Read the model definition and answer for the solid it produces. Units are mm, in the model's axes. A direction names the side the tool comes from. Coordinates: 2 decimals unless noted, no trailing zeros. Write each loop counter-clockwise with the first axis right and the second up, starting at its lowest first coordinate (ties: lowest second). Pieces come first, ordered by that corner, then holes.
(1) Section A-A on y = -30.5 is taken. Write down the section's boundary in (x, z) (3 decimals).
(2) Given pin 1 (2 mm diameter, centred on y = 16, z = 15.5, fed in from +X); pin 2 (4 mm diameter, centred on x = -27.5, y = -8.5, fed in from +Z); pin 3 (5 mm diameter, centred on y = -14.5, z = -34, fed in from +X); pin 4 (21 mm diameter, centred on y = 8.5, z = -7.5, fed in from -X) (3 decimals), each flat-ended and moving along its own axis, determine where each tip first touches the part or whether it passes through.
(3) Which of the six approach directions +Z, -Z, +X, -X, +Y, -Y give full straight-line access (tool end or side, diameter ignored) to faces 5 (the cylindrical face through (20.882, -32.56, 13.314)), 6 (the cylindrical face through (-32.56, 13.314, 20.882)), 7 (the cylindrical face through (6.33, -20.11, -40.27))?
(4) Find the intervals of material crossed by probe 1 along X at (y, z) = (0, -39.5) (3 decimals); probe 2 along X at (y, z) = (0, -16.25) (3 decimals), in increasing order.
(5) The mould has two halves that part along X. Classify faces 1 (the conical face through (-20.755, -58.745, -4.609)), 2 (the cylindrical face through (-40.27, 20.11, 6.33)), 3 (the flat face through (16, 3, -20.955)), 4 (the cylindrical face through (10.73, 11.7, -12.95)): +X half, -X half, draft (parallel to the pull), parting line (faces both ways), or undercut.
from build123d import *


with BuildPart() as f3:
    # F0 (on Right) → F3 (revolve)
    with BuildSketch(Plane.YZ):
        with BuildLine():
            Line((-52.6758568757, 24.765), (-59.055, 21.082))
            Line((-59.055, 21.082), (-20.955, 21.082))
            Line((-20.955, 21.082), (-20.955, 15.875))
            Line((-20.955, 15.875), (0, 15.875))
            ThreePointArc((0, 15.875), (11.2253201513, 11.2253201513), (15.875, 0))
            Line((15.875, 0), (24.765, 0))
            ThreePointArc((24.765, 0), (17.5114994361, 17.5114994361), (0, 24.765))
            Line((0, 24.765), (-52.6758568757, 24.765))
        make_face()
        with BuildLine():
            Line((-20.955, 21.082), (-59.055, 21.082))
            Line((-59.055, 21.082), (-59.055, 0))
            Line((-59.055, 0), (0, 0))
            Line((0, 0), (10.5189766587, 0))
            Line((10.5189766587, 0), (15.875, 0))
            ThreePointArc((15.875, 0), (11.2253201513, 11.2253201513), (0, 15.875))
            Line((0, 15.875), (-20.955, 15.875))
            Line((-20.955, 15.875), (-20.955, 21.082))
        make_face()
    revolve(axis=Axis((0, -21.59, 0), (0, 1, 0)))

    # F1 (on Right) → F4 (revolve)
    with BuildSketch(Plane.YZ):
        with BuildLine():
            Line((-24.765, -52.6758568757), (-21.082, -59.055))
            Line((-21.082, -59.055), (-21.082, -20.955))
            Line((-21.082, -20.955), (-15.875, -20.955))
            Line((-15.875, -20.955), (-15.875, 0))
            ThreePointArc((-15.875, 0), (-11.2253201513, 11.2253201513), (0, 15.875))
            Line((0, 15.875), (0, 24.765))
            ThreePointArc((0, 24.765), (-17.5114994361, 17.5114994361), (-24.765, 0))
            Line((-24.765, 0), (-24.765, -52.6758568757))
        make_face()
        with BuildLine():
            Line((-21.082, -20.955), (-21.082, -59.055))
            Line((-21.082, -59.055), (0, -59.055))
            Line((0, -59.055), (0, 0))
            Line((0, 0), (0, 15.875))
            ThreePointArc((0, 15.875), (-11.2253201513, 11.2253201513), (-15.875, 0))
            Line((-15.875, 0), (-15.875, -20.955))
            Line((-15.875, -20.955), (-21.082, -20.955))
        make_face()
    revolve(axis=Axis((0, 0, -21.59), (0, 0, 1)))

    # F2 (on Top) → F5 (revolve)
    with BuildSketch(Plane.XY):
        with BuildLine():
            Line((-52.6758568757, 24.765), (-59.055, 21.082))
            Line((-59.055, 21.082), (-20.955, 21.082))
            Line((-20.955, 21.082), (-20.955, 15.875))
            Line((-20.955, 15.875), (0, 15.875))
            ThreePointArc((0, 15.875), (11.2253201513, 11.2253201513), (15.875, 0))
            Line((15.875, 0), (24.765, 0))
            ThreePointArc((24.765, 0), (17.5114994361, 17.5114994361), (0, 24.765))
            Line((0, 24.765), (-52.6758568757, 24.765))
        make_face()
        with BuildLine():
            Line((-20.955, 21.082), (-59.055, 21.082))
            Line((-59.055, 21.082), (-59.055, 0))
            Line((-59.055, 0), (-12.5608257832, 0))
            Line((-12.5608257832, 0), (0, 0))
            Line((0, 0), (15.875, 0))
            ThreePointArc((15.875, 0), (11.2253201513, 11.2253201513), (0, 15.875))
            Line((0, 15.875), (-20.955, 15.875))
            Line((-20.955, 15.875), (-20.955, 21.082))
        make_face()
    revolve(axis=Axis((-21.59, 0, 0), (1, 0, 0)))

    # F0 (on Right) → F6 (revolve, cut)
    with BuildSketch(Plane.YZ):
        with BuildLine():
            Line((-20.955, 21.082), (-59.055, 21.082))
            Line((-59.055, 21.082), (-59.055, 0))
            Line((-59.055, 0), (0, 0))
            Line((0, 0), (10.5189766587, 0))
            Line((10.5189766587, 0), (15.875, 0))
            ThreePointArc((15.875, 0), (11.2253201513, 11.2253201513), (0, 15.875))
            Line((0, 15.875), (-20.955, 15.875))
            Line((-20.955, 15.875), (-20.955, 21.082))
        make_face()
    revolve(axis=Axis((0, -21.59, 0), (0, 1, 0)), mode=Mode.SUBTRACT)

    # F1 (on Right) → F7 (revolve, cut)
    with BuildSketch(Plane.YZ):
        with BuildLine():
            Line((-21.082, -20.955), (-21.082, -59.055))
            Line((-21.082, -59.055), (0, -59.055))
            Line((0, -59.055), (0, 0))
            Line((0, 0), (0, 15.875))
            ThreePointArc((0, 15.875), (-11.2253201513, 11.2253201513), (-15.875, 0))
            Line((-15.875, 0), (-15.875, -20.955))
            Line((-15.875, -20.955), (-21.082, -20.955))
        make_face()
    revolve(axis=Axis((0, 0, -21.59), (0, 0, 1)), mode=Mode.SUBTRACT)

    # F2 (on Top) → F8 (revolve, cut)
    with BuildSketch(Plane.XY):
        with BuildLine():
            Line((-20.955, 21.082), (-59.055, 21.082))
            Line((-59.055, 21.082), (-59.055, 0))
            Line((-59.055, 0), (-12.5608257832, 0))
            Line((-12.5608257832, 0), (0, 0))
            Line((0, 0), (15.875, 0))
            ThreePointArc((15.875, 0), (11.2253201513, 11.2253201513), (0, 15.875))
            Line((0, 15.875), (-20.955, 15.875))
            Line((-20.955, 15.875), (-20.955, 21.082))
        make_face()
    revolve(axis=Axis((-21.59, 0, 0), (1, 0, 0)), mode=Mode.SUBTRACT)


solid = f3.part
Response:
1. outline: circle Ø49.53 at (0, 0); hole circle Ø42.164 at (0, 0)
2. pin 1: stops at x = 12.67
2. pin 2: stops at z = 23.9
2. pin 3: stops at x = 21.66
2. pin 4: stops at x = -59.055
3. face 5: -Y
3. face 6: -X
3. face 7: -Z
4. probe 1: x = -24.765 to -21.082, 21.082 to 24.765
4. probe 2: x = -20.955 to -15.875, 15.875 to 24.765
5. face 1: parting line
5. face 2: draft
5. face 3: undercut
5. face 4: undercut
